```python
from build123d import *

# Parameters (mm, degrees)
SKETCH1_R               = 1.575
BOSS_EXTRUDE1_DEPTH     = 12.5
SKETCH2_W               = 13.385271969
SKETCH2_H               = 10
CUT_EXTRUDE1_DEPTH      = 36
SKETCH3_R               = 1.75
CUT_EXTRUDE2_DEPTH      = 25
SKETCH4_R               = 4
CUT_EXTRUDE3_DEPTH      = 4
FILLET1_R               = 2
SKETCH5_R               = 2
CUT_EXTRUDE4_DEPTH      = 10
SKETCH7_R               = 3.575
CUT_EXTRUDE5_DEPTH      = 3.5
SKETCH8_R               = 10
CUT_EXTRUDE6_DEPTH      = 5
CUT_EXTRUDE6_DEPTH_BACK = 5
CUT_EXTRUDE7_DEPTH      = 3


with BuildPart() as part:
    # Sketch1 → Boss-Extrude1 (new body, symmetric)
    with BuildSketch(Plane(origin=(0, 0, 0), x_dir=(1, 0, 0), z_dir=(0, 1, 0))):
        Polygon((0, 0), (-43.5, 0), (-56.885271969, -10.457720596), (-56.885271969, -21.057720596), (-48.596177418, -32.057720596), (-43.5, -35), (-37, -35), (-37, -10), (0, -10), align=None)
        with Locations((-48.5, -17.5)):
            Circle(SKETCH1_R, mode=Mode.SUBTRACT)
    extrude(amount=BOSS_EXTRUDE1_DEPTH, both=True)

    # Sketch2 → Cut-Extrude1 (cut, through all)
    with BuildSketch(Plane.XY.offset(35)):
        with Locations((-50.192635985, 0)):
            Rectangle(SKETCH2_W, SKETCH2_H)
    extrude(amount=-CUT_EXTRUDE1_DEPTH, mode=Mode.SUBTRACT)

    # Sketch3 → Cut-Extrude2 (cut)
    with BuildSketch(Plane.XY.offset(10)):
        with Locations((-27, 0)):
            Circle(SKETCH3_R)
        with Locations((-7, 0)):
            Circle(SKETCH3_R)
    extrude(amount=-CUT_EXTRUDE2_DEPTH, mode=Mode.SUBTRACT)

    # Sketch4 → Cut-Extrude3 (cut)
    with BuildSketch(Plane(origin=(0, 0, 0), x_dir=(-1, 0, 0), z_dir=(0, 0, -1))):
        with Locations((7, 0)):
            Circle(SKETCH4_R)
        with Locations((27, 0)):
            Circle(SKETCH4_R)
    extrude(amount=-CUT_EXTRUDE3_DEPTH, mode=Mode.SUBTRACT)

    # Fillet1
    fillet1_edges = [part.edges().sort_by_distance(p)[0] for p in [
        (-56.885271969, 8.75, 21.057720596),
        (-56.885271969, 8.75, 10.457720596),
        (0, 0, 0),
        (-56.885271969, -8.75, 21.057720596),
        (-56.885271969, -8.75, 10.457720596),
    ]]
    fillet(fillet1_edges, radius=FILLET1_R)

    # Sketch5 → Cut-Extrude4 (cut)
    with BuildSketch(Plane.ZY.offset(43.5)):
        with Locations((30, 0)):
            Circle(SKETCH5_R)
    extrude(amount=-CUT_EXTRUDE4_DEPTH, mode=Mode.SUBTRACT)

    # Sketch7 → Cut-Extrude5 (cut)
    with BuildSketch(Plane.ZY.offset(43.5)):
        with Locations((30, 0)):
            Circle(SKETCH7_R)
    extrude(amount=-CUT_EXTRUDE5_DEPTH, mode=Mode.SUBTRACT)

    # Sketch8 → Cut-Extrude6 (cut, two sides)
    with BuildSketch(Plane(origin=(0, 0, 0), x_dir=(1, 0, 0), z_dir=(0, 1, 0))) as cut_extrude6_sk:
        with Locations((-48.5, -17.5)):
            Circle(SKETCH8_R)
    extrude(amount=CUT_EXTRUDE6_DEPTH, mode=Mode.SUBTRACT)
    extrude(cut_extrude6_sk.sketch, amount=-CUT_EXTRUDE6_DEPTH_BACK, mode=Mode.SUBTRACT)

    # Sketch9 → Cut-Extrude7 (cut)
    with BuildSketch(Plane.XZ.offset(12.5)):
        Polygon((-46.800589834, 14.481390206), (-45.036102151, 17.462427479), (-46.735512318, 20.481037272), (-50.199410166, 20.518609794), (-51.963897849, 17.537572521), (-50.264487682, 14.518962728), align=None)
    extrude(amount=-CUT_EXTRUDE7_DEPTH, mode=Mode.SUBTRACT)


solid = part.part
```
Part model, mm, in its own coordinate system. A direction names the side the tool comes from. Give positions to 0.01 mm unless a question says otherwise; leave off trailing zeros. Write each loop counter-clockwise with the first axis right and the second up, starting at its lowest first coordinate (ties: lowest second). Pieces come first, ordered by that corner, then holes. Notation, with made-up numbers: (10.25, 70) -> (17.25, 70) arc R31 cw to (17.25, 107) -> close; hole circle Ø7 at (67, 66.25). An arc over 180 degrees is marked (long way). Put each result on its own line as item: value. Start each with the question number.
Item 1: Which spindle directions (+Z, -Z, +X, -X, +Y, -Y) get a long thin tool onto all of the face, cutting with end or side? Do faces 4 (the face through (-37, 0, 23)), 5 (the face through (-46, -5, 18)), 6 (the face through (-50.1, -9.5, 18.2)). Say none if no direction does.
Item 2: Pull direction X, two halves, no side cores. Call faces 1 (the face through (-41.77, 0.16, 26.43)), 2 (the face through (-23.8, -2.4, 2)), 3 (the face through (-56.785, 8.802, 21.015)): pulls with the +X half, pulls with the -X half, needs draft (parallel to the pull), parting line crosses it, or undercut.
Item 3: Cut at C-C (z = 16.5). List the corners of the cut face in (x, y), then the cut area to 3 significant figures.
Item 4: Cut at B-B (x = -7). List the corners of the cut face in (y, z).
Item 5: Cut at D-D (z = 30). List the corners of the cut face in (x, y) (3 decimals), then the cut area to 3 significant figures.
Item 6: Pin check, flat tips, straight feed: pin 1 Ø6.5 at (x, y) = (-7, 0) entering from +Z; pin 2 Ø4 at (y, z) = (8.5, 28) entering from +X; pin 3 Ø8 at (y, z) = (0, 30) entering from -X. Stop position of each tip, or through.
Item 7: Cut at A-A (y = 0). State how many separate pieces and enclosed holes the cut face has, then the cut area to 3 significant figures.
Item 8: Wall check: L1, parallel to Y at x = -27, z = 8.15; L2, parallel to Y at x = -50, z = 14; L3, parallel to Z at x = -15.5, y = -7.5. Give the ranges that are in metal, low to high. Write a range as [from, to].
Answer list:
1. face 4: +Z, +X, +Y, -Y
1. face 5: -X
1. face 6: -Y
2. face 1: needs draft
2. face 2: undercut
2. face 3: pulls with the -X half
3. outline: (-56.89, -12.5) -> (-51.38, -12.5) -> (-51.38, -9.5) -> (-49.72, -9.5) -> (-49.72, -5) -> (-56.89, -5) -> close; (-56.89, 5) -> (-49.72, 5) -> (-49.72, 12.5) -> (-56.89, 12.5) -> close; (-47.28, -9.5) -> (-45.61, -9.5) -> (-45.61, -12.5) -> (-37, -12.5) -> (-37, 12.5) -> (-47.28, 12.5) -> (-47.28, 5) -> (-38.55, 5) -> (-38.55, -5) -> (-47.28, -5) -> close
3. area: 267 mm2
4. outline: (-12.5, 0) -> (-4, 0) -> (-4, 4) -> (-1.75, 4) -> (-1.75, 10) -> (-12.5, 10) -> close; (1.75, 4) -> (4, 4) -> (4, 0) -> (12.5, 0) -> (12.5, 10) -> (1.75, 10) -> close
5. outline: (-50.147, -12.5) -> (-37, -12.5) -> (-37, -2) -> (-40, -2) -> (-40, -3.575) -> (-43.5, -3.575) -> (-43.5, -5) -> (-50.147, -5) -> close; (-50.147, 5) -> (-43.5, 5) -> (-43.5, 3.575) -> (-40, 3.575) -> (-40, 2) -> (-37, 2) -> (-37, 12.5) -> (-50.147, 12.5) -> close
5. area: 225 mm2
6. pin 1: stops at z = 10
6. pin 2: stops at x = -37
6. pin 3: stops at x = -43.5
7. separate pieces: 4
7. enclosed holes: 0
7. area: 392 mm2
8. L1: y = [-12.5, -1.75], [1.75, 12.5]
8. L2: y = [-12.5, -5], [5, 12.5]
8. L3: z = [0, 10]
